from build123d import *

# Parameters (mm, degrees)
F0_W      = 40.64
F0_H      = 25.4
F1_DEPTH  = 17.78
F2_DEPTH  = 25.4
F3_W      = 25.4
F3_H      = 40.64
F4_DEPTH  = 17.78
F5_W      = 40.64
F5_H      = 17.78
F6_DEPTH  = 50.8
F7_W      = 25.4
F7_H      = 40.64
F8_DEPTH  = 25.4
F9_W      = 40.64
F9_H      = 25.4
F10_DEPTH = 58.42
F12_DEPTH = 17.78


with BuildPart() as f1:
    # F0 (on Right) → F1 (new body)
    with BuildSketch(Plane.YZ):
        with Locations((36.7695213166, 12.7)):
            Rectangle(F0_W, F0_H)
    extrude(amount=F1_DEPTH)

    # F2 (add): a face of the model
    f2_faces = [f1.faces().sort_by_distance(p)[0] for p in [
        (0, 36.7695213166, 12.7),
    ]]
    extrude(f2_faces, amount=F2_DEPTH)

    # F3 (on face) → F4 (join)
    with BuildSketch(Plane.XY.offset(25.4)):
        with Locations((-12.7, 36.7695213166)):
            Rectangle(F3_W, F3_H)
    extrude(amount=F4_DEPTH)

    # F5 (on face) → F6 (join)
    with BuildSketch(Plane(origin=(-25.4, 0, 0), x_dir=(0, -1, 0), z_dir=(-1, 0, 0))):
        with Locations((-36.7695213166, 34.29)):
            Rectangle(F5_W, F5_H)
    extrude(amount=F6_DEPTH)

    # F7 (on face) → F8 (join)
    with BuildSketch(Plane(origin=(0, 0, 25.4), x_dir=(1, 0, 0), z_dir=(0, 0, -1))):
        with Locations((-63.5, -36.7695213166)):
            Rectangle(F7_W, F7_H)
    extrude(amount=F8_DEPTH)

    # F9 (on face) → F10 (join)
    with BuildSketch(Plane(origin=(-76.2, 0, 0), x_dir=(0, -1, 0), z_dir=(-1, 0, 0))):
        with Locations((-36.7695213166, 12.7)):
            Rectangle(F9_W, F9_H)
    extrude(amount=F10_DEPTH)

    # F11 (on face) → F12 (join)
    with BuildSketch(Plane.XZ.offset(-16.4495213166)):
        Polygon((-76.2, 25.4), (-116.84, 25.4), (-116.84, 0), (-50.8, 0), (-50.8, 25.4), align=None)
    extrude(amount=F12_DEPTH)


solid = f1.part
Design review of the part built by this model. Coordinates are the model's own, in mm. A direction names the side the tool comes from. Coordinates: 2 decimals unless noted, no trailing zeros. Loops run counter-clockwise (first coordinate to the right, second up) from the corner with the lowest first, then second, coordinate; pieces in that order, holes last. Notation, with made-up numbers: M -18,21 L 2,21 A23 cw 2,35 Z; hole C 37,30 d6. An arc over 180 degrees is marked long. Answer as CSV lines item,"result".
Item 1: Machinability: for faces 4 (the face through (-76.2, 37, 34)), 5 (the face through (-29, 16.45, 26)), 6 (the face through (-50.8, 28, 13)), which of the approach directions +Z, -Z, +X, -X, +Y, -Y give a long, thin tool a straight path to every point of the face, cutting with its end or side? Answer none if there is none.
Answer list:
face 4,"+Z, -X, +Y, -Y"
face 5,"+Z, +X, -Y"
face 6,"-Z, +Y, -Y"
Item 2: The part is to be moulded in two halves that separate along X. For faces 1 (the face through (-134.62, 37, 13)), 2 (the face through (-38, 37, 25.4)), 3 (the face through (-38, 37, 43.18)), say which applies: pulls with the +X half, pulls with the -X half, needs draft (parallel to the pull), parting line crosses it, or undercut.
Answer list:
face 1,"pulls with the -X half"
face 2,"undercut"
face 3,"needs draft"
Item 3: Add section A-A on z = 15.5. State the section outline as (x, y) points.
Answer list:
outline,"M -134.62,16.45 L -116.84,16.45 L -116.84,-1.33 L -50.8,-1.33 L -50.8,57.09 L -134.62,57.09 Z; M -25.4,16.45 L 17.78,16.45 L 17.78,57.09 L -25.4,57.09 Z"
Item 4: For probe 1 along X at (y, z) = (19, 10); probe 2 along X at (y, z) = (45.5, 36.5); probe 3 along Z at (x, y) = (-40, 29), list the stretches that pass through material, from the lowest coordinate up.
Answer list:
probe 1,"-134.62 to -50.8, -25.4 to 17.78"
probe 2,"-76.2 to 0"
probe 3,"25.4 to 43.18"
Item 5: Add section B-B on y = 26. State the section outline as (x, z) points, plus the area to 3 significant figures.
Answer list:
outline,"M -134.62,0 L -50.8,0 L -50.8,25.4 L -25.4,25.4 L -25.4,0 L 17.78,0 L 17.78,25.4 L 0,25.4 L 0,43.18 L -76.2,43.18 L -76.2,25.4 L -134.62,25.4 Z"
area,"4,580 mm²"
Item 6: Add section D-D on z = 36. State the section outline as (x, y) points.
Answer list:
outline,"M -76.2,16.45 L 0,16.45 L 0,57.09 L -76.2,57.09 Z"
Item 7: Add section C-C on x = -63.5. State the section outline as (y, z) points.
Answer list:
outline,"M -1.33,0 L 57.09,0 L 57.09,43.18 L 16.45,43.18 L 16.45,25.4 L -1.33,25.4 Z"
Item 8: For P1, Ø12, axis at y = 18.5, z = 33.5, coming from the +X side; P2, Ø6, axis at x = -100, y = 37.5, coming from the +Z side; P3, Ø7.5, axis at x = -41.5, y = 40.5, coming from the -Z side, all flat-tipped, find the tip position at first contact; note any pin that passes through.
Answer list:
P1,"x = 0"
P2,"z = 25.4"
P3,"z = 25.4"
